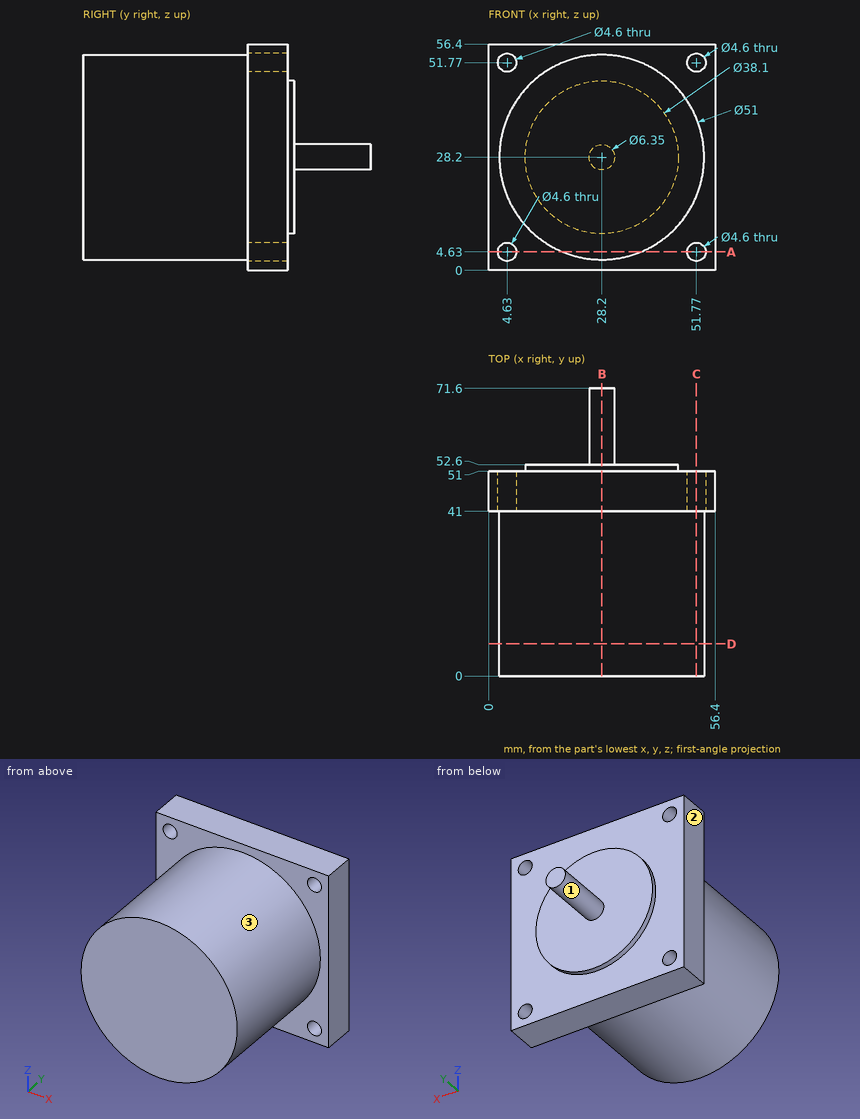
Check sheet for the drawn part. Datum: minimum x, y, z corner. Units: mm. A direction names the side the tool comes from. Round coordinates to 2 decimals unless told otherwise and drop trailing zeros. Order: outer loops, then holes, each group sorted by start corner. A loop starts at its lowest first (then second) coordinate and runs counter-clockwise, first axis right, second up. Notation, with made-up numbers: (27, -16) -> (86, -16) arc R18 cw to (86, -6) -> close; hole circle Ø1 at (8, 26.5). An arc over 180 degrees is marked (long way). Put each result on its own line as item: value. Start each with the question number.
(1) Section check C-C (x = 51.77). Enter the section's corners in (y, z).
(2) Depth check by flat-ended pin: pin 1 Ø5 at (y, z) = (23, 26) entering from +X; pin 2 Ø6 at (x, y) = (42.5, 26) entering from -Z; pin 3 Ø1 at (x, z) = (18, 17) entering from +Y. Enter the tip coordinate at first touch or a pass-through.
(3) Section check B-B (x = 28.2). Enter the section's corners in (y, z) (3 decimals), then the cut area to 3 significant figures.
(4) Section check D-D (y = 8). Enter the section's corners in (x, z), then the cut area to 3 significant figures.
(5) Section check A-A (z = 4.63). Enter the section's corners in (x, y), then the cut area to 3 significant figures.
(6) Material ranges on line 1 along Z through (x, y) = (4.63, 44.75); line 2 along X through (y, z) = (47, 4), recorded low to high.
(7) Tool access check on the marked faces 1, 2 and 3. Record the directions out of +Z, -Z, +X, -X, +Y, -Y that give a thin tool (end or side, any length) a straight path to the whole face; none if there is none.
Completed:
1. outline: (0, 18.47) -> (41, 18.47) -> (41, 6.93) -> (51, 6.93) -> (51, 49.47) -> (41, 49.47) -> (41, 37.93) -> (0, 37.93) -> close; (41, 0) -> (51, 0) -> (51, 2.33) -> (41, 2.33) -> close; (41, 54.07) -> (51, 54.07) -> (51, 56.4) -> (41, 56.4) -> close
2. pin 1: stops at x = 53.7
2. pin 2: stops at z = 5.34
2. pin 3: stops at y = 52.6
3. outline: (0, 2.7) -> (41, 2.7) -> (41, 0) -> (51, 0) -> (51, 9.15) -> (52.6, 9.15) -> (52.6, 25.025) -> (71.6, 25.025) -> (71.6, 31.375) -> (52.6, 31.375) -> (52.6, 47.25) -> (51, 47.25) -> (51, 56.4) -> (41, 56.4) -> (41, 53.7) -> (0, 53.7) -> close
3. area: 2,840 mm2
4. outline: circle Ø51 at (28.2, 28.2)
4. area: 2,040 mm2
5. outline: (0, 41) -> (2.33, 41) -> (2.33, 51) -> (0, 51) -> close; (6.93, 41) -> (18.47, 41) -> (18.47, 0) -> (37.93, 0) -> (37.93, 41) -> (49.47, 41) -> (49.47, 51) -> (6.93, 51) -> close; (54.07, 41) -> (56.4, 41) -> (56.4, 51) -> (54.07, 51) -> close
5. area: 1,270 mm2
6. line 1: z = 0 to 2.33, 6.93 to 49.47, 54.07 to 56.4
6. line 2: x = 0 to 2.42, 6.84 to 49.56, 53.98 to 56.4
7. face 1: +Y
7. face 2: +Z, -Z, -X, +Y, -Y
7. face 3: -Y
